For this review, take the finished solid that the model builds, in its own axes (mm). A direction names the side the tool comes from. Coordinates: 2 decimals unless noted, no trailing zeros. Order: outer loops, then holes, each group sorted by start corner. A loop starts at its lowest first (then second) coordinate and runs counter-clockwise, first axis right, second up. Notation, with made-up numbers: (3.5, 32) -> (42.5, 32) arc R31 cw to (42.5, 56) -> close; hole circle Ø9 at (11.25, 45). An arc over 180 degrees is marked (long way). Return JSON: item names as keys, results as strings. Group by question number.
Item 1: Insertion check: pin 1 (1 mm diameter, centred on x = 284.5, z = 4.5, fed in from -Y); pin 2 (17.5 mm diameter, centred on x = 290, y = 144, fed in from +Z) (3 decimals); pin 3 (11 mm diameter, centred on x = 290.5, y = 67.5, fed in from -Z). Each pin has a flat end and moves straight along its axis. Give the tip position at first contact, or say it passes through.
Item 2: Take a section at D-D (y = 137). Write out the cut boundary in (x, z), then the cut area to 3 significant figures.
Item 3: Take a section at A-A (x = 290). Write out the cut boundary in (y, z).
Item 4: Take a section at C-C (z = 3.75). Write out the cut boundary in (x, y), then the cut area to 3 significant figures.
Item 5: Draft analysis for pull direction Y (two halves, no side actions). For faces 1 (the flat face through (270, 91, 3)), 2 (the cylindrical face through (290, 123, 3)), 3 (the cylindrical face through (290, 19, 3)), state which applies: +Y half, -Y half, draft (parallel to the pull), parting line (faces both ways), or undercut.
Item 6: Take a section at B-B (y = 75.5). Write out the cut boundary in (x, z), then the cut area to 3 significant figures.
Item 7: Machinability: for faces 4 (the cylindrical face through (290, 164, 3)), 5 (the flat face through (290, 76, 6)), which of the approach directions +Z, -Z, +X, -X, +Y, -Y give a long, thin tool a straight path to every point of the face, cutting with its end or side? Answer none if there is none.
Item 8: For line 1 along X through (y, z) = (54, 1); line 2 along Y through (x, z) = (287.5, 1.5); line 3 along Y through (x, z) = (290, 2.75), list the stretches that pass through material, from the lowest coordinate up.
Autodesk Inventor part; units mm, degrees
ref_plane "YZ Plane" through (0, 0, 0) normal (1, 0, 0) x (0, 1, 0)
ref_plane "XZ Plane" through (0, 0, 0) normal (0, 1, 0) x (-1, 0, 0)
ref_plane "XY Plane" through (0, 0, 0) normal (0, 0, 1) x (1, 0, 0)
sketch "Sketch1" plane through (0, 0, 0) normal (0, 0, 1) x (1, 0, 0)
  line L0 (0, 0) -> (220, 0) construction
  line L1 (220, 0) -> (220, 9) construction
  line L2 (220, 9) -> (0, 9) construction
  line L3 (0, 9) -> (0, 0) construction
  line L4 (0, 9) -> (90.94, 295.0593) construction
  line L5 (129.06, 295.0593) -> (220, 9) construction
  circle A0 centre (110, 289) radius 11 construction
  line L6 (96.1101, 281.616) -> (103.5522, 305.0259) construction
  arc A1 (129.06, 295.0593) -> (90.94, 295.0593) centre (110, 289) ccw construction
  line L7 (99, 275.5567) -> (99, 269.1274) construction
  line L8 (110, 289) -> (110, 144) construction
  line L9 (130, 289) -> (130, 144) construction
  line L10 (90, 144) -> (90, 289) construction
  arc A2 (130, 289) -> (90, 289) centre (110, 289) ccw construction
  arc A3 (90, 144) -> (130, 144) centre (110, 144) ccw construction
  line L11 (290, 144) -> (290, 249) construction
  line L12 (310, 144) -> (310, 249) construction
  line L13 (270, 249) -> (270, 144) construction
  arc A4 (270, 144) -> (310, 144) centre (290, 144) ccw construction
  arc A5 (310, 249) -> (270, 249) centre (290, 249) ccw construction
  arc A6 (90, 289) -> (130, 289) centre (110, 289) ccw construction
  line L14 (98.9216, 269) -> (121.0784, 269) construction
  line L15 (209.0249, 269) -> (370.9751, 269) construction
  line L16 (209.0249, 144) -> (370.9751, 144) construction
  line L17 (290, 144) -> (290, 39) construction
  line L18 (310, 144) -> (310, 39)
  line L19 (270, 39) -> (270, 144)
  arc A7 (310, 144) -> (270, 144) centre (290, 144) ccw
  arc A8 (270, 39) -> (310, 39) centre (290, 39) ccw
  line L20 (209.0249, 19) -> (370.9751, 19) construction
  circle A9 centre (110, 289) radius 11 construction
  circle A10 centre (110, 144) radius 11 construction
  circle A11 centre (290, 144) radius 11
  circle A12 centre (290, 39) radius 11
  line L21 (290, 39) -> (290, 112) construction
  line L22 (301, 39) -> (301, 112)
  line L23 (279, 112) -> (279, 39)
  arc A13 (279, 39) -> (301, 39) centre (290, 39) ccw
  arc A14 (301, 112) -> (279, 112) centre (290, 112) ccw
  line L24 (290, 123) -> (290, 133) construction
  point P0 (110, 0)
  point P1 (110, 216.5)
  point P2 (110, 309)
  point P3 (290, 196.5)
  point P4 (110, 269)
  point P5 (110, 269)
  point P6 (290, 269)
  point P7 (290, 75.5)
  dimension "d18" = 22
  dimension "d0" = 9
  dimension "d1" = 220
  dimension "d2" = 22
  dimension "d3" = 280
  dimension "d4" = 9
  dimension "d7" = 40
  dimension "d8" = 40
  dimension "pendgap" = 0
  dimension "abovethefloor" = 10
  dimension "d11" = 105
  dimension "d12" = 145
  dimension "d14" = 22
  dimension "d19" = 22
  dimension "d20" = 50
  dimension "d23" = 10
extrude "Extrusion3" add sketch "Sketch1" along normal blind 7 contours L18 A8 L19 A7 | A12 | A12 L23 A14 L22
extrude "Extrusion4" cut sketch "Sketch1" along normal blind 6 contours A11 | A12 | A12 L23 A14 L22
properties part number "DBP-3-pendulum2"
Findings below:
{
 "1": {"pin 1": "stops at y = 19.64", "pin 2": "passes through", "pin 3": "stops at z = 6"},
 "2": {"outline": "(270, 0) -> (281.51, 0) -> (281.51, 7) -> (270, 7) -> close; (298.49, 0) -> (310, 0) -> (310, 7) -> (298.49, 7) -> close", "area": "161 mm2"},
 "3": {"outline": "(19, 0) -> (28, 0) -> (28, 6) -> (123, 6) -> (123, 0) -> (133, 0) -> (133, 7) -> (19, 7) -> close; (155, 0) -> (164, 0) -> (164, 7) -> (155, 7) -> close"},
 "4": {"outline": "(270, 39) arc R20 ccw to (310, 39) -> (310, 144) arc R20 ccw to (270, 144) -> close; hole (279, 39) arc R11 ccw to (301, 39) -> (301, 112) arc R11 ccw to (279, 112) -> close; hole circle Ø22 at (290, 144)", "area": "3,090 mm2"},
 "5": {"face 1": "draft", "face 2": "undercut", "face 3": "-Y half"},
 "6": {"outline": "(270, 0) -> (279, 0) -> (279, 6) -> (301, 6) -> (301, 0) -> (310, 0) -> (310, 7) -> (270, 7) -> close", "area": "148 mm2"},
 "7": {"face 4": "+Z, -Z, +Y", "face 5": "-Z"},
 "8": {"line 1": "x = 270 to 279, 301 to 310", "line 2": "y = 19.16 to 28.29, 122.71 to 133.29, 154.71 to 163.84", "line 3": "y = 19 to 28, 123 to 133, 155 to 164"}
}
